Read the model definition and answer for the solid it produces. Units are mm, in the model's axes. Face numbers are marked on the shaded views. A direction names the side the tool comes from. Coordinates: 2 decimals unless noted, no trailing zeros. Order: outer loops, then holes, each group sorted by start corner. A loop starts at its lowest first (then second) coordinate and runs counter-clockwise, first axis right, second up. Notation, with made-up numbers: M 53.25,64.5 L 86.25,64.5 A22 ccw 86.25,78.5 Z; hole C 60.5,57 d8. An arc over 180 degrees is marked long. Write each question's results on one line, items separated by ' | '.
Autodesk Inventor part; units mm, degrees
ref_plane "YZ Plane" through (0, 0, 0) normal (1, 0, 0) x (0, 1, 0)
ref_plane "XZ Plane" through (0, 0, 0) normal (0, 1, 0) x (-1, 0, 0)
ref_plane "XY Plane" through (0, 0, 0) normal (0, 0, 1) x (1, 0, 0)
sketch "Sketch1" plane through (0, 0, 0) normal (0, 0, 1) x (1, 0, 0)
  line L0 (9.525, -6.35) -> (-9.525, -6.35)
  line L1 (-9.525, -6.35) -> (-9.525, 6.35)
  line L2 (-9.525, 6.35) -> (9.525, 6.35)
  line L3 (9.525, 6.35) -> (9.525, -6.35)
  line L4 (9.525, -6.35) -> (-9.525, 6.35) construction
  line L5 (-9.525, -6.35) -> (9.525, 6.35) construction
  point P0 (0, 0)
  dimension "d0" = 19.05
  dimension "d1" = 12.7
extrude "Extrusion1" add sketch "Sketch1" along normal blind 6.35
sketch "Sketch2" plane through (0, 0, 6.35) normal (0, 0, 1) x (1, 0, 0)
  line L0 (9.525, 6.35) -> (-9.525, 6.35)
  line L1 (-9.525, 6.35) -> (-9.525, -6.35)
  line L2 (-9.525, -6.35) -> (9.525, -6.35)
  line L3 (9.525, -6.35) -> (9.525, 6.35)
  line L4 (9.525, -4.445) -> (-9.525, -4.445)
  line L5 (-9.525, -4.445) -> (-9.525, 4.445)
  line L6 (-9.525, 4.445) -> (9.525, 4.445)
  line L7 (9.525, 4.445) -> (9.525, -4.445)
  line L8 (9.525, -4.445) -> (-9.525, 4.445) construction
  line L9 (-9.525, -4.445) -> (9.525, 4.445) construction
  point P0 (0, 0)
  dimension "d4" = 19.05
  dimension "d5" = 8.89
extrude "Extrusion2" add sketch "Sketch2" along normal blind 6.35 contours L3 L4 L1 L6
sketch "Sketch3" plane through (9.525, -6.35, 0) normal (1, 0, 0) x (0, 0, -1)
  line L0 (0, 0) -> (0, 12.7)
  line L1 (0, 12.7) -> (-6.35, 12.7)
  line L2 (-6.35, 10.795) -> (-6.35, 12.7)
  line L3 (-6.35, 10.795) -> (-12.7, 10.795)
  line L4 (-12.7, 1.905) -> (-12.7, 10.795)
  line L5 (-6.35, 1.905) -> (-12.7, 1.905)
  line L6 (-6.35, 0) -> (-6.35, 1.905)
  line L7 (0, 0) -> (-6.35, 0)
  line L8 (-6.35, 12.7) -> (-6.35, 10.795) construction
  line L9 (-6.35, 10.795) -> (-6.35, 1.905) construction
  line L10 (-12.7, 6.35) -> (0, 6.35) construction
  line L11 (-9.525, 10.795) -> (-9.525, 1.905) construction
  line L12 (-6.35, 1.905) -> (-12.7, 1.905) construction
  circle A0 centre (-9.525, 6.35) radius 1.651
  dimension "d8" = 3.302
extrude "Extrusion3" cut sketch "Sketch3" against normal through all contours A0
fillet "Fillet1" radius 3.175 4 edges at (0, 4.445, 12.7) (0, -4.445, 12.7) (0, 6.35, 6.35) (0, -6.35, 6.35)
properties part number "Torsion_Spring_Mounts"
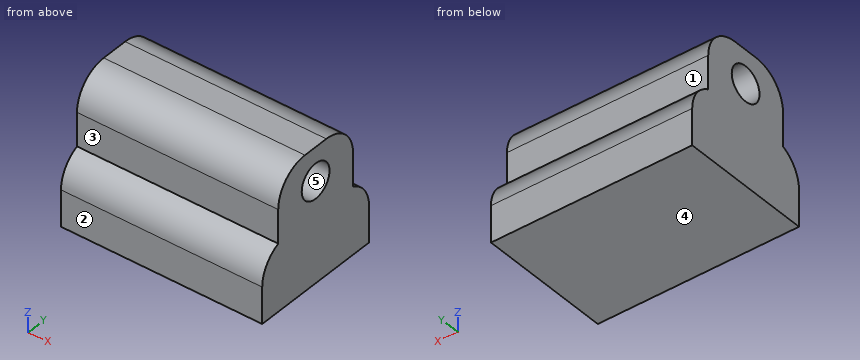
(1) For the marked faces 1 and 2, determine the directions among +Z, -Z, +X, -X, +Y, -Y from which every point of the face is accessible in a straight line to the end or side of a thin tool.
Conclusion:
face 1: +Z, +X, -X, +Y | face 2: +Z, -Z, +X, -X, -Y
(2) The part is cut by section C-C, the plane z = 10.5. Write down the section's boundary in (x, y) (3 decimals).
Conclusion:
outline: M -9.525,-4.292 L 9.525,-4.292 L 9.525,-1.332 L -9.525,-1.332 Z; M -9.525,1.332 L 9.525,1.332 L 9.525,4.292 L -9.525,4.292 Z
(3) Straight lines are drawn through the part: line 1 (Z direction, x = -7.75, y = -1.5); line 2 (Y direction, x = 6.25, z = 7.75) (3 decimals); line 3 (Y direction, x = 4.75, z = 9) (3 decimals). For each, find the intervals that lie inside material, in ascending order.
Conclusion:
line 1: 0 to 8.84, 10.21 to 12.69 | line 2: -4.445 to 4.445 | line 3: -4.445 to -1.565, 1.565 to 4.445
(4) The part is cut by section B-B, the plane x = 2.25. Write down the section's boundary in (y, z) (3 decimals), then the cut area to 3 significant figures.
Conclusion:
outline: M -6.35,0 L 6.35,0 L 6.35,3.44 A3.175 ccw 4.445,6.35 L 4.445,9.525 A3.175 ccw 1.27,12.7 L -1.27,12.7 A3.175 ccw -4.445,9.525 L -4.445,6.35 A3.175 ccw -6.35,3.44 Z; hole C 0,9.525 d3.302 | area: 121 mm²
(5) The part is cut by section A-A, the plane y = 0. Write down the section's boundary in (x, z) (3 decimals), then the cut area to 3 significant figures.
Conclusion:
outline: M -9.525,0 L 9.525,0 L 9.525,7.874 L -9.525,7.874 Z; M -9.525,11.176 L 9.525,11.176 L 9.525,12.7 L -9.525,12.7 Z | area: 179 mm²
(6) Given pin 1 (1.6 mm diameter, centred on x = 0, z = 8, fed in from -Y) (3 decimals); pin 2 (3.5 mm diameter, centred on x = 4.5, z = 8, fed in from +Y), each flat-ended and moving along its own axis, determine where each tip first touches the part or whether it passes through.
Conclusion:
pin 1: y = -4.445 | pin 2: y = 4.65
(7) The mould has two halves that part along Z. Classify the marked faces 3, 4 and 5: pulls with the +Z half, pulls with the -Z half, needs draft (parallel to the pull), parting line crosses it, or undercut.
Conclusion:
face 3: needs draft | face 4: pulls with the -Z half | face 5: undercut
(8) The part is cut by section D-D, the plane y = -3.5. Write down the section's boundary in (x, z) (3 decimals).
Conclusion:
outline: M -9.525,0 L 9.525,0 L 9.525,11.785 L -9.525,11.785 Z
